from build123d import *

# Parameters (mm, degrees)
SKETCH1_R             = 2
BOSS_EXTRUDE1_DEPTH   = 5
BOSS_EXTRUDE1_2_DEPTH = 5
BOSS_EXTRUDE1_3_DEPTH = 5
BOSS_EXTRUDE1_4_DEPTH = 5
SKETCH3_W             = 38.1
SKETCH3_H             = 25.4
BOSS_EXTRUDE2_DEPTH   = 10
SKETCH4_W             = 25.4
SKETCH4_H             = 17.78
BOSS_EXTRUDE3_DEPTH   = 2
SKETCH2_R             = 1.25
CUT_EXTRUDE1_DEPTH    = 10
SKETCH6_W             = 5.998216144
SKETCH6_H             = 2
CUT_EXTRUDE3_DEPTH    = 2
SKETCH7_W             = 6
SKETCH7_H             = 2
CUT_EXTRUDE4_DEPTH    = 2
SKETCH8_W             = 68.1
SKETCH8_H             = 20
BOSS_EXTRUDE4_DEPTH   = 5
SKETCH9_R             = 3.175
CUT_EXTRUDE5_DEPTH    = 5
FILLET1_R             = 2


with BuildPart() as part:
    # Sketch1 → Boss-Extrude1 (new body)
    with BuildSketch(Plane(origin=(0, 0, 0), x_dir=(1, 0, 0), z_dir=(0, 1, 0))):
        with Locations(Location((-10.16, 6.35, 0), (0, 0, 270))):
            Circle(SKETCH1_R)
    extrude(amount=BOSS_EXTRUDE1_DEPTH)



with BuildPart() as body_2:
    # Sketch1 → Boss-Extrude1 2 (new body)
    with BuildSketch(Plane(origin=(0, 0, 0), x_dir=(1, 0, 0), z_dir=(0, 1, 0))):
        with Locations(Location((10.16, 6.35, 0), (0, 0, 270))):
            Circle(SKETCH1_R)
    extrude(amount=BOSS_EXTRUDE1_2_DEPTH)


with BuildPart() as body_3:
    # Sketch1 → Boss-Extrude1 3 (new body)
    with BuildSketch(Plane(origin=(0, 0, 0), x_dir=(1, 0, 0), z_dir=(0, 1, 0))):
        with Locations(Location((10.16, -6.35, 0), (0, 0, 270))):
            Circle(SKETCH1_R)
    extrude(amount=BOSS_EXTRUDE1_3_DEPTH)


with BuildPart() as body_4:
    # Sketch1 → Boss-Extrude1 4 (new body)
    with BuildSketch(Plane(origin=(0, 0, 0), x_dir=(1, 0, 0), z_dir=(0, 1, 0))):
        with Locations(Location((-10.16, -6.35, 0), (0, 0, 270))):
            Circle(SKETCH1_R)
    extrude(amount=BOSS_EXTRUDE1_4_DEPTH)


with BuildPart() as part_1:
    add(part.part)

    add(body_2.part)  # Boss-Extrude2 merges body 2

    add(body_3.part)  # Boss-Extrude2 merges body 3

    add(body_4.part)  # Boss-Extrude2 merges body 4
    # Sketch3 → Boss-Extrude2 (add)
    with BuildSketch(Plane.XZ):
        Rectangle(SKETCH3_W, SKETCH3_H)
    extrude(amount=BOSS_EXTRUDE2_DEPTH)

    # Sketch4 → Boss-Extrude3 (add)
    with BuildSketch(Plane(origin=(0, 0, 0), x_dir=(1, 0, 0), z_dir=(0, 1, 0))):
        Rectangle(SKETCH4_W, SKETCH4_H)
    extrude(amount=BOSS_EXTRUDE3_DEPTH)

    # Sketch2 → Cut-Extrude1 (cut)
    with BuildSketch(Plane(origin=(0, 5, 0), x_dir=(1, 0, 0), z_dir=(0, 1, 0))):
        with Locations(Location((-10.16, 6.35, 0), (0, 0, 270))):
            Circle(SKETCH2_R)
        with Locations(Location((10.16, 6.35, 0), (0, 0, 270))):
            Circle(SKETCH2_R)
        with Locations(Location((10.16, -6.35, 0), (0, 0, 270))):
            Circle(SKETCH2_R)
        with Locations(Location((-10.16, -6.35, 0), (0, 0, 270))):
            Circle(SKETCH2_R)
    extrude(amount=-CUT_EXTRUDE1_DEPTH, mode=Mode.SUBTRACT)

    # Sketch6 → Cut-Extrude3 (cut)
    with BuildSketch(Plane(origin=(0, 0, -12.7), x_dir=(-1, 0, 0), z_dir=(0, 0, -1))):
        with Locations((0, -1)):
            Rectangle(SKETCH6_W, SKETCH6_H)
    cut_extrude3 = extrude(amount=-CUT_EXTRUDE3_DEPTH, mode=Mode.SUBTRACT)

    # Mirror1: Cut-Extrude3 across plane
    add(cut_extrude3.mirror(Plane.XY), mode=Mode.SUBTRACT)

    # Sketch7 → Cut-Extrude4 (cut)
    with BuildSketch(Plane.ZY.offset(19.05)):
        with Locations((0.00303896, -1)):
            Rectangle(SKETCH7_W, SKETCH7_H)
    cut_extrude4 = extrude(amount=-CUT_EXTRUDE4_DEPTH, mode=Mode.SUBTRACT)

    # Mirror2: Cut-Extrude4 across plane
    add(cut_extrude4.mirror(Plane(origin=(0, 0, 0), x_dir=(0, 0, 1), z_dir=(1, 0, 0))), mode=Mode.SUBTRACT)

    # Sketch8 → Boss-Extrude4 (add)
    with BuildSketch(Plane(origin=(0, 0, -12.7), x_dir=(-1, 0, 0), z_dir=(0, 0, -1))):
        with Locations((0, -5)):
            Rectangle(SKETCH8_W, SKETCH8_H)
    extrude(amount=BOSS_EXTRUDE4_DEPTH)

    # Sketch9 → Cut-Extrude5 (cut)
    with BuildSketch(Plane.XY.offset(-12.7)):
        with Locations((-26.55, -5)):
            Circle(SKETCH9_R)
        with Locations((26.55, -5)):
            Circle(SKETCH9_R)
    extrude(amount=-CUT_EXTRUDE5_DEPTH, mode=Mode.SUBTRACT)

    # Fillet1
    fillet1_edges = [part_1.edges().sort_by_distance(p)[0] for p in [
        (-19.05, -5, 12.7),
        (-19.05, -5, -12.7),
        (19.05, -5, -12.7),
        (19.05, -5, 12.7),
        (-19.05, -10, 0),
        (0, -10, -12.7),
        (19.05, -10, 0),
        (0, -10, 12.7),
    ]]
    fillet(fillet1_edges, radius=FILLET1_R)


solid = part_1.part
Here's how the part is built. I have some questions about the finished solid (model axes, mm). A direction names the side the tool comes from. Round coordinates to 2 decimals unless told otherwise and drop trailing zeros. Loops run counter-clockwise (first coordinate to the right, second up) from the corner with the lowest first, then second, coordinate; pieces in that order, holes last. Notation, with made-up numbers: M 30,3 L 88,3 A13 cw 88,16 Z; hole C 81.25,-29 d3. An arc over 180 degrees is marked long. Write each question's results on one line, items separated by ' | '. Start each with the question number.
(1) Thinking about a two-plate mould opening in Z: for faces 1 (the flat face through (0, -5, -17.7)), 2 (the flat face through (0, -1, -10.7)), 3 (the cylindrical face through (23.38, -4.86, -15.16)), which applies, pulls with the +Z half, pulls with the -Z half, needs draft (parallel to the pull), parting line crosses it, or undercut?
(2) I want a section at D-D (x = 26.55). Please give me the cut outline in (y, z) (3 decimals).
(3) I want a section at A-A (y = 0.75). Please give me the cut outline in (x, z).
(4) Will these pins go through, and if not, where does the flat tip stop? P1, Ø2, axis at y = -1.5, z = -1, coming from the -X side; P2, Ø1.6, axis at y = -1.5, z = 12, coming from the +X side; P3, Ø7.5, axis at x = -26.55, y = -5, coming from the +Z side.
(5) I want a section at C-C (x = -7.5). Please give me the cut outline in (y, z).
(6) If I drill on probe 1 along X at (y, z) = (1.25, 6.35); probe 2 along X at (y, z) = (-1, 6.35); probe 3 along X at (y, z) = (2.5, -6.35), over which ranges is the centre line in solid material (lowest first)? Write a range as from..to.
(7) I want a section at B-B (y = -4.25). Please give me the cut outline in (x, z).
(8) On a 3-axis mill with a long thin cutter (end or side, diameter ignored), from which of +Z, -Z, +X, -X, +Y, -Y can I reach the whole of each face in a straight line? I mean faces 4 (the flat face through (0, -10, 0)), 5 (the flat face through (2.999, -1, 12)), 6 (the flat face through (-18, -2, 0)), 7 (the flat face through (0, 1, 8.89)), 8 (the cylindrical face through (8.208, 3.479, 5.916)). Say none if no direction works.
Solved:
1) face 1: pulls with the -Z half | face 2: undercut | face 3: needs draft
2) outline: M -15,-17.7 L -8.175,-17.7 L -8.175,-12.7 L -15,-12.7 Z; M -1.825,-17.7 L 5,-17.7 L 5,-12.7 L -1.825,-12.7 Z
3) outline: M -34.05,-17.7 L 34.05,-17.7 L 34.05,-12.7 L -34.05,-12.7 Z; M -12.7,-8.89 L 12.7,-8.89 L 12.7,8.89 L -12.7,8.89 Z; hole C -10.16,-6.35 d2.5; hole C -10.16,6.35 d2.5; hole C 10.16,-6.35 d2.5; hole C 10.16,6.35 d2.5
4) P1: stops at x = -19.05 | P2: stops at x = 18.99 | P3: stops at z = -12.7
5) outline: M -15,-17.7 L 5,-17.7 L 5,-12.7 L 0,-12.7 L 0,-8.89 L 2,-8.89 L 2,8.89 L 0,8.89 L 0,12.7 L -8,12.7 A2 ccw -10,10.7 L -10,-10.7 A2 cw -12,-12.7 L -15,-12.7 Z
6) probe 1: x = -12.7..-11.41, -8.91..8.91, 11.41..12.7 | probe 2: x = -19.05..-11.41, -8.91..8.91, 11.41..19.05 | probe 3: x = -12.16..-11.41, -8.91..-8.16, 8.16..8.91, 11.41..12.16
7) outline: M -34.05,-17.7 L -29.64,-17.7 L -29.64,-12.7 L -34.05,-12.7 Z; M -23.46,-17.7 L 23.46,-17.7 L 23.46,-12.7 L 21.05,-12.7 A2 cw 19.05,-10.7 L 19.05,10.7 A2 ccw 17.05,12.7 L -17.05,12.7 A2 ccw -19.05,10.7 L -19.05,-10.7 A2 cw -21.05,-12.7 L -23.46,-12.7 Z; M 29.64,-17.7 L 34.05,-17.7 L 34.05,-12.7 L 29.64,-12.7 Z; hole C -10.16,-6.35 d2.5; hole C -10.16,6.35 d2.5; hole C 10.16,-6.35 d2.5; hole C 10.16,6.35 d2.5
8) face 4: +Z, +X, -X, -Y | face 5: +Z, +Y | face 6: -X, +Y | face 7: +Z, +X, -X, +Y | face 8: +Y
